Input: part model. Units: mm. Frame: model coordinates. Face numbers are marked on the shaded views. Give positions to 0.01 mm unless a question says otherwise; leave off trailing zeros. Write each loop counter-clockwise with the first axis right and the second up, starting at its lowest first coordinate (ties: lowest second). Pieces come first, ordered by that corner, then holes. Notation, with made-up numbers: (-28, 36.5) - (-22, 36.5) arc R10 ccw to (-22, 40.5) - close; hole circle Ø4 at (62.25, 59.5). An arc over 180 degrees is marked (long way). Answer as a JSON object with one key per item and string values. Group by question number.
Autodesk Inventor part; units mm, degrees
ref_plane "YZ Plane" through (0, 0, 0) normal (1, 0, 0) x (0, 1, 0)
ref_plane "XZ Plane" through (0, 0, 0) normal (0, 1, 0) x (-1, 0, 0)
ref_plane "XY Plane" through (0, 0, 0) normal (0, 0, 1) x (1, 0, 0)
sketch "Sketch1" plane through (0, 0, 0) normal (0, 0, 1) x (1, 0, 0)
  line L0 (-18.75, 15) -> (18.75, 15)
  line L1 (18.75, 15) -> (18.75, -15)
  line L2 (18.75, -15) -> (-18.75, -15)
  line L3 (-18.75, -15) -> (-18.75, 15)
  line L4 (-18.75, 15) -> (18.75, -15) construction
  line L5 (18.75, 15) -> (-18.75, -15) construction
  line L6 (18.75, 0) -> (1.25, 0)
  circle A0 centre (1.25, 0) radius 7.6
  circle A1 centre (1.25, 0) radius 12
  line L7 (-11.25, 12.5) -> (13.75, 12.5)
  line L8 (13.75, 12.5) -> (13.75, -12.5)
  line L9 (13.75, -12.5) -> (-11.25, -12.5)
  line L10 (-11.25, -12.5) -> (-11.25, 12.5)
  line L11 (-11.25, 12.5) -> (13.75, -12.5) construction
  line L12 (13.75, 12.5) -> (-11.25, -12.5) construction
  line L13 (13.75, 12.5) -> (-11.25, -12.5)
  circle A2 centre (9.7353, 8.4853) radius 1.75
  circle A3 centre (-7.2353, 8.4853) radius 1.75
  circle A4 centre (-7.2353, -8.4853) radius 1.75
  circle A5 centre (9.7353, -8.4853) radius 1.75
  point P0 (0, 0)
  dimension "d4" = 24
  dimension "d0" = 37.5
  dimension "d1" = 30
  dimension "d2" = 17.5
  dimension "d3" = 15.2
  dimension "d5" = 25
  dimension "d6" = 25
  dimension "d7" = 3.5
  dimension "d10" = 360
extrude "Extrusion1" add sketch "Sketch1" along normal blind 10 contours L8 L9 L13 A4 A1 A5 L6 | L6 A1 A2 L13 L8 | L0 L1 L2 L3 | A1 A5 A4 L13 A0 L6 | L6 A0 L13 A2 A1 | L13 A2 A1 A3 A4 L10 L7 | A0 L13 A4 A1 A3 A2
properties part number "POSIBLE CORTE"
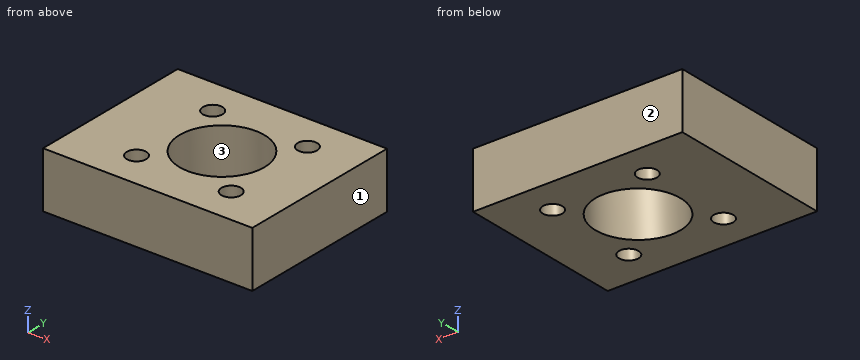
1) Cut plane A-A on x = 1.25. Return the cut outline in (y, z), and give its area (3 significant figures).
2) Line query: line 1 along X through (y, z) = (0, 7.25); line 2 along X through (y, z) = (-8.5, 1.25); line 3 along Y through (x, z) = (1.25, 2.25). Output: solid intervals per line, ascending. Write a range as from..to.
3) Cut plane C-C on z = 1.5. Return the cut outline in (x, y).
4) Cut plane D-D on y = 9. Return the cut outline in (x, z), and give its area (3 significant figures).
5) Mould query, pull axis Y, two halves, no side actions, for the marked faces 1, 2 and 3. Classes: +Y half, -Y half, draft (parallel to the pull), parting line (faces both ways), or undercut.
6) Cut plane B-B on y = 0. Return the cut outline in (x, z).
Filled in:
{
 "1": {"outline": "(-15, 0) - (-7.6, 0) - (-7.6, 10) - (-15, 10) - close; (7.6, 0) - (15, 0) - (15, 10) - (7.6, 10) - close", "area": "148 mm²"},
 "2": {"line 1": "x = -18.75..-6.35, 8.85..18.75", "line 2": "x = -18.75..-8.99, -5.49..7.99, 11.49..18.75", "line 3": "y = -15..-7.6, 7.6..15"},
 "3": {"outline": "(-18.75, -15) - (18.75, -15) - (18.75, 15) - (-18.75, 15) - close; hole circle Ø3.5 at (-7.24, -8.49); hole circle Ø3.5 at (-7.24, 8.49); hole circle Ø15.2 at (1.25, 0); hole circle Ø3.5 at (9.74, -8.49); hole circle Ø3.5 at (9.74, 8.49)"},
 "4": {"outline": "(-18.75, 0) - (-8.91, 0) - (-8.91, 10) - (-18.75, 10) - close; (-5.56, 0) - (8.06, 0) - (8.06, 10) - (-5.56, 10) - close; (11.41, 0) - (18.75, 0) - (18.75, 10) - (11.41, 10) - close", "area": "308 mm²"},
 "5": {"face 1": "draft", "face 2": "+Y half", "face 3": "undercut"},
 "6": {"outline": "(-18.75, 0) - (-6.35, 0) - (-6.35, 10) - (-18.75, 10) - close; (8.85, 0) - (18.75, 0) - (18.75, 10) - (8.85, 10) - close"}
}
